from build123d import *

# Parameters (mm, degrees)
SKETCH_1_R               = 15
EXTRUDE_1_DEPTH          = 160
SKETCH_2_OUTSIDE_W       = 65.106
SKETCH_2_OUTSIDE_H       = 65.106
SKETCH_2_OUTSIDE_R       = 12.5
CUT_EXTRUDE_1_DEPTH      = 92
SKETCH_3_OUTSIDE_W       = 65.106
SKETCH_3_OUTSIDE_H       = 65.106
SKETCH_3_OUTSIDE_R       = 12.5
CUT_EXTRUDE_2_DEPTH      = 63
CHAMFER_1_SIZE           = 1
CUT_EXTRUDE_START        = 12.5
CUT_EXTRUDE_3_DEPTH      = 4
HOLE_WIZARD_M121_D       = 10.2
HOLE_WIZARD_M121_DEPTH   = 32.75
HOLE_WIZARD_M121_TIP     = 2.944486373
CHAMFER_2_SIZE           = 1
CUT_EXTRUDE_4_DEPTH      = 16
CUT_EXTRUDE_4_DEPTH_BACK = 16
SKETCH_9_R               = 15
SKETCH_9_R_2             = 11.9
CUT_EXTRUDE_5_DEPTH      = 1.3
SKETCH_10_R              = 15
SKETCH_10_R_2            = 12.5
CUT_EXTRUDE_6_DEPTH      = 7.3


with BuildPart() as part:
    # Эскиз1 → Бобышка-Вытянуть1 (new body)
    with BuildSketch(Plane(origin=(0, 0, 0), x_dir=(0, 0, -1), z_dir=(1, 0, 0))):
        Circle(SKETCH_1_R)
    extrude(amount=EXTRUDE_1_DEPTH)

    # Эскиз2 outside → Вырез-Вытянуть1 (cut)
    with BuildSketch(Plane.ZY):
        Rectangle(SKETCH_2_OUTSIDE_W, SKETCH_2_OUTSIDE_H)
        Circle(SKETCH_2_OUTSIDE_R, mode=Mode.SUBTRACT)
    extrude(amount=-CUT_EXTRUDE_1_DEPTH, mode=Mode.SUBTRACT)

    # Эскиз3 outside → Вырез-Вытянуть2 (cut)
    with BuildSketch(Plane(origin=(160, 0, 0), x_dir=(0, 0, -1), z_dir=(1, 0, 0))):
        Rectangle(SKETCH_3_OUTSIDE_W, SKETCH_3_OUTSIDE_H)
        Circle(SKETCH_3_OUTSIDE_R, mode=Mode.SUBTRACT)
    extrude(amount=-CUT_EXTRUDE_2_DEPTH, mode=Mode.SUBTRACT)

    # Фаска1
    chamfer_1_edges = [part.edges().sort_by_distance(p)[0] for p in [
        (0, 0, -12.5),
        (97, 0, 15),
        (160, 0, 12.5),
        (92, 0, 15),
    ]]
    chamfer(chamfer_1_edges, length=CHAMFER_1_SIZE)

    # Эскиз4 → Вырез-Вытянуть3 (cut)
    with BuildSketch(Plane(origin=(0, 0, 0), x_dir=(1, 0, 0), z_dir=(0, 1, 0)).offset(CUT_EXTRUDE_START)):
        with BuildLine():
            Line((10, 4), (22.2, 4))
            ThreePointArc((22.2, 4), (26.2, 0), (22.2, -4))
            Line((22.2, -4), (10, -4))
            ThreePointArc((10, -4), (6, 0), (10, 4))
        make_face()
        with BuildLine():
            Line((70, 4), (82.2, 4))
            ThreePointArc((82.2, 4), (86.2, 0), (82.2, -4))
            Line((82.2, -4), (70, -4))
            ThreePointArc((70, -4), (66, 0), (70, 4))
        make_face()
    extrude(amount=-CUT_EXTRUDE_3_DEPTH, mode=Mode.SUBTRACT)

    # Отверстие обработанное метчиком M121
    with Locations(Plane.ZY):
        with Locations((0, 0)):
            Hole(HOLE_WIZARD_M121_D / 2, depth=HOLE_WIZARD_M121_DEPTH)
            with Locations((0, 0, -(HOLE_WIZARD_M121_DEPTH + HOLE_WIZARD_M121_TIP / 2))):  # 120° drill point
                Cone(0, HOLE_WIZARD_M121_D / 2, HOLE_WIZARD_M121_TIP, mode=Mode.SUBTRACT)

    # Фаска2
    chamfer_2_edges = [part.edges().sort_by_distance(p)[0] for p in [
        (0, 0, 5.1),
    ]]
    chamfer(chamfer_2_edges, length=CHAMFER_2_SIZE)

    # Эскиз8 → Вырез-Вытянуть4 (cut, two sides)
    with BuildSketch(Plane(origin=(0, 0, 0), x_dir=(1, 0, 0), z_dir=(0, 1, 0))) as cut_extrude_4_sk:
        with BuildLine():
            Line((147.5, -5.5), (117.5, -5.5))
            ThreePointArc((117.5, -5.5), (112, 0), (117.5, 5.5))
            Line((117.5, 5.5), (147.5, 5.5))
            ThreePointArc((147.5, 5.5), (153, 0), (147.5, -5.5))
        make_face()
    extrude(amount=CUT_EXTRUDE_4_DEPTH, mode=Mode.SUBTRACT)
    extrude(cut_extrude_4_sk.sketch, amount=-CUT_EXTRUDE_4_DEPTH_BACK, mode=Mode.SUBTRACT)

    # Эскиз9 → Вырез-Вытянуть5 (cut)
    with BuildSketch(Plane.ZY.offset(-92)):
        Circle(SKETCH_9_R)
        Circle(SKETCH_9_R_2, mode=Mode.SUBTRACT)
    extrude(amount=-CUT_EXTRUDE_5_DEPTH, mode=Mode.SUBTRACT)

    # Эскиз10 → Вырез-Вытянуть6 (cut)
    with BuildSketch(Plane(origin=(97, 0, 0), x_dir=(0, 0, -1), z_dir=(1, 0, 0))):
        Circle(SKETCH_10_R)
        Circle(SKETCH_10_R_2, mode=Mode.SUBTRACT)
    extrude(amount=-CUT_EXTRUDE_6_DEPTH, mode=Mode.SUBTRACT)


solid = part.part
Design review of the part built by this model. Coordinates are the model's own, in mm. A direction names the side the tool comes from. Round coordinates to 2 decimals unless told otherwise and drop trailing zeros.
Item 1: For pin 1 Ø4 at (x, y) = (16.5, 3) entering from -Z; pin 2 Ø1 at (x, y) = (17, 10) entering from +Z; pin 3 Ø4 at (x, z) = (15.5, 1.5) entering from +Y; pin 4 Ø5 at (y, z) = (1.5, 8.5) entering from -X, all flat-tipped, find the tip position at first contact; note any pin that passes through.
Item 2: Wall thickness on L1, parallel to Y at x = 24, z = 0; L2, parallel to Y at x = 26.5, z = 0; L3, parallel to Z at x = 139.5, y = 1: over which ranges is each line inside the solid? List them lowest first.
Item 3: For faces 1 (the flat face through (76, 10, 4)), 2 (the flat face through (92, -5, 11)), 3 (the flat face through (133, 0, 5.5)), list the 3-axis set-ups (+Z, -Z, +X, -X, +Y, -Y) from which the entire face can be reached by the end or side of a thin tool; tool diameter is ignored.
Check values:
1. pin 1: stops at z = -12.46
1. pin 2: stops at z = 8.12
1. pin 3: stops at y = 8.5
1. pin 4: stops at x = 0
2. L1: y = -12.5 to -5.1, 5.1 to 8.5
2. L2: y = -12.5 to -5.1, 5.1 to 12.5
2. L3: z = -12.46 to -5.5, 5.5 to 12.46
3. face 1: +Y
3. face 2: none
3. face 3: +Y, -Y
